```python
from build123d import *

# Parameters (mm, degrees)
SKETCH1_W           = 939.8
SKETCH1_H           = 330.2
BOSS_EXTRUDE1_DEPTH = 101.6
FILLET1_R           = 152.4
SHELL1_T            = -6.35
SKETCH3_W           = 135.128
SKETCH3_H           = 43.18
CUT_EXTRUDE1_DEPTH  = 127.762


with BuildPart() as part:
    # Sketch1 → Boss-Extrude1 (new body)
    with BuildSketch(Plane(origin=(0, 0, 0), x_dir=(1, 0, 0), z_dir=(0, 1, 0))):
        with Locations((469.9, 165.1)):
            Rectangle(SKETCH1_W, SKETCH1_H)
    extrude(amount=BOSS_EXTRUDE1_DEPTH)

    # Fillet1
    # the kernel refuses this fillet: 152.4 mm, written as the material it takes off along each edge
    with BuildSketch(Plane(origin=(0, 101.6, -689.410244843), x_dir=(0, -1, 0), z_dir=(0, 0, 1))) as fillet1_piece_1:
        with BuildLine():
            CenterArc((152.4, 143.684097937), FILLET1_R, 180, 70.528779366)
            Line((0, 143.684097937), (-3.048, 143.684097937))
            Line((-3.048, 143.684097937), (-3.048, 0))
            Line((-3.048, 0), (0, -3.048))
            ThreePointArc((0, -3.048), (50.8, -3.048), (100.584, -2.873681959))
            Line((100.584, -2.873681959), (101.6, 0))
        make_face()
    extrude(amount=1048.620489686, mode=Mode.SUBTRACT)

    # Shell1
    shell1_openings = [part.faces().sort_by_distance(p)[0] for p in [
        (469.9, 0, -165.1),
    ]]
    offset(amount=SHELL1_T, openings=shell1_openings, kind=Kind.INTERSECTION)

    # Sketch3 → Cut-Extrude1 (cut)
    with BuildSketch(Plane(origin=(0, 101.6, 0), x_dir=(1, 0, 0), z_dir=(0, 1, 0))):
        with Locations((517.285069024, 49.525)):
            Rectangle(SKETCH3_W, SKETCH3_H)
        with Locations((827.165069024, 280.675)):
            Rectangle(SKETCH3_W, SKETCH3_H)
        with Locations((827.165069024, 49.525)):
            Rectangle(SKETCH3_W, SKETCH3_H)
        with Locations((517.285069024, 280.675)):
            Rectangle(SKETCH3_W, SKETCH3_H)
        with Locations((211.248097937, 280.67)):
            Rectangle(SKETCH3_W, SKETCH3_H)
        with Locations((211.248097937, 49.53)):
            Rectangle(SKETCH3_W, SKETCH3_H)
    extrude(amount=-CUT_EXTRUDE1_DEPTH, mode=Mode.SUBTRACT)


solid = part.part
```
For this review, take the finished solid that the model builds, in its own axes (mm). A direction names the side the tool comes from. Coordinates: 2 decimals unless noted, no trailing zeros. Order: outer loops, then holes, each group sorted by start corner. A loop starts at its lowest first (then second) coordinate and runs counter-clockwise, first axis right, second up. Notation, with made-up numbers: (-20.5, -38.5) - (38.5, -38.5) arc R18 cw to (38.5, -19.5) - close; hole circle Ø10 at (41.5, 31). An arc over 180 degrees is marked (long way). Answer as a JSON object with one key per item and string values. Group by question number.
1. Clearance check with flat-ended pins moving along their axes: P1, Ø1.5, axis at y = 16, z = -295, coming from the -X side; P2, Ø1.5, axis at y = 85.5, z = -44, coming from the -X side; P3, Ø4, axis at y = 19, z = -61.5, coming from the -X side. State where each tip first meets the part, or that it passes through.
2. We need section A-A on x = 515. State the section outline as (y, z) points (3 decimals), then the cut area to 3 significant figures.
3. We need section B-B on z = -57.5. State the section outline as (x, y) points, then the cut area to 3 significant figures.
4. For faces 1 (the flat face through (463, 50, 0)), 2 (the cylindrical face through (61.307, 69.801, -167.322)), list the 3-axis set-ups (+Z, -Z, +X, -X, +Y, -Y) from which the entire face can be reached by the end or side of a thin tool; tool diameter is ignored.
5. For probe 1 along Z at (x, y) = (215, 4.5); probe 2 along X at (y, z) = (38, -226.5), list the stretches that pass through material, from the lowest coordinate up.
6. The part is to be moulded in two halves that separate along Z. For faces 3 (the flat face through (933.45, 47, -163)), 4 (the flat face through (463, 50, -330.2)), 5 (the flat face through (468, 0, -325)), say which applies: pulls with the +Z half, pulls with the -Z half, needs draft (parallel to the pull), parting line crosses it, or undercut.
7. We need section D-D on x = 736. State the section outline as (y, z) points, then the cut area to 3 significant figures.
8. We need section C-C on y = 36.5. State the section outline as (x, z) points, then the cut area to 3 significant figures.
Final values:
{
 "1": {"P1": "x = 6.34", "P2": "x = 74.03", "P3": "x = 7.2"},
 "2": {"outline": "(0, -330.2) - (101.6, -330.2) - (101.6, -302.265) - (95.25, -302.265) - (95.25, -323.85) - (0, -323.85) - close; (0, -6.35) - (95.25, -6.35) - (95.25, -27.935) - (101.6, -27.935) - (101.6, 0) - (0, 0) - close; (95.25, -259.085) - (101.6, -259.085) - (101.6, -71.115) - (95.25, -71.115) - close", "area": "2,760 mm²"},
 "3": {"outline": "(0, 0) - (6.75, 0) arc R146.05 cw to (143.68, 95.25) - (143.68, 101.6) arc R152.4 ccw to start; (278.81, 95.25) - (449.72, 95.25) - (449.72, 101.6) - (278.81, 101.6) - close; (584.85, 95.25) - (759.6, 95.25) - (759.6, 101.6) - (584.85, 101.6) - close; (894.73, 95.25) - (933.45, 95.25) - (933.45, 0) - (939.8, 0) - (939.8, 101.6) - (894.73, 101.6) - close", "area": "4,250 mm²"},
 "4": {"face 1": "+Z, +X, -X, +Y, -Y", "face 2": "-Y"},
 "5": {"probe 1": "-330.2 to -323.85, -6.35 to 0", "probe 2": "19.83 to 27.73, 933.45 to 939.8"},
 "6": {"face 3": "undercut", "face 4": "pulls with the -Z half", "face 5": "needs draft"},
 "7": {"outline": "(0, -330.2) - (101.6, -330.2) - (101.6, 0) - (0, 0) - (0, -6.35) - (95.25, -6.35) - (95.25, -323.85) - (0, -323.85) - close", "area": "3,310 mm²"},
 "8": {"outline": "(18.77, -330.2) - (939.8, -330.2) - (939.8, 0) - (18.77, 0) - close; hole (26.6, -323.85) - (933.45, -323.85) - (933.45, -6.35) - (26.6, -6.35) - close", "area": "16,200 mm²"}
}
